Geometry: final body of the model. Coordinates: model frame, mm. Face numbers are marked on the shaded views. A direction names the side the tool comes from. Give positions to 0.01 mm unless a question says otherwise; leave off trailing zeros. Loops run counter-clockwise (first coordinate to the right, second up) from the corner with the lowest first, then second, coordinate; pieces in that order, holes last. Notation, with made-up numbers: (19, 83) -> (68, 83) arc R30 cw to (68, 111) -> close; hole circle Ø4 at (52, 2.25). An arc over 180 degrees is marked (long way). Answer in a Markdown table with one row per item. Add a question column.
1) Draft query along X for the marked faces 1, 2 and 3. Return one class per face: +X half, -X half, draft (parallel to the pull), parting line (faces both ways), or undercut.
2) Line query: line 1 (Y direction, x = 36.5, z = -34); line 2 (X direction, y = -4.5, z = -15); line 3 (Y direction, x = -7.5, z = 29.5). Output: solid intervals per line, ascending. Write a range as from..to.
3) Access query for the marked faces 4, 5 and 6. Directions: +Z, -Z, +X, -X, +Y, -Y. A direction counts if a zero-diameter tool reaches every point of the face in a straight line with its end or side. Return the directions, or none.
4) Section query D-D (x = -52.5). Give the number of separate pieces and of enclosed holes in the cut face, plus the area to 3 significant figures.
5) Section query A-A (z = 21). Return the cut outline in (x, y), plus the area to 3 significant figures.
6) Section query B-B (y = 0). Return the cut outline in (x, z), plus the area to 3 significant figures.
7) Section query C-C (x = 45.5). Return the cut outline in (y, z), plus the area to 3 significant figures.
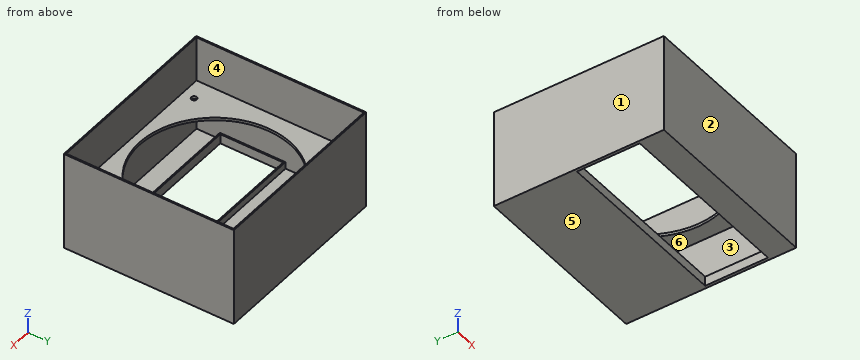
```python
from build123d import *

# Parameters (mm, degrees)
F0_W     = 134
F0_H     = 122
F0_R     = 2
F0_R_2   = 55
F1_DEPTH = 2
F0_W_2   = 136
F0_H_2   = 124
F2_DEPTH = 35
F3_W     = 136
F3_H     = 124
F3_W_2   = 134
F3_H_2   = 122
F3_W_3   = 133.8
F3_H_3   = 47.8
F3_W_4   = 131.8
F3_H_4   = 45.8
F4_DEPTH = 2
F5_DEPTH = 5


with BuildPart() as f1:
    # F0 (on Top) → F1 (new body)
    with BuildSketch(Plane.XY):
        Rectangle(F0_W, F0_H)
        with Locations((-52.5, -52.5)):
            Circle(F0_R, mode=Mode.SUBTRACT)
        with Locations((52.5, -52.5)):
            Circle(F0_R, mode=Mode.SUBTRACT)
        with Locations((-52.5, 52.5)):
            Circle(F0_R, mode=Mode.SUBTRACT)
        Circle(F0_R_2, mode=Mode.SUBTRACT)
        with Locations((52.5, 52.5)):
            Circle(F0_R, mode=Mode.SUBTRACT)
    extrude(amount=F1_DEPTH)

    # F0 (on Top) → F2 (join, symmetric)
    with BuildSketch(Plane.XY):
        Rectangle(F0_W_2, F0_H_2)
        Rectangle(F0_W, F0_H, mode=Mode.SUBTRACT)
    extrude(amount=F2_DEPTH, both=True)

    # F3 (on face) → F4 (join)
    with BuildSketch(Plane(origin=(0, 0, -35), x_dir=(1, 0, 0), z_dir=(0, 0, -1))):
        Rectangle(F3_W, F3_H)
        Rectangle(F3_W_2, F3_H_2, mode=Mode.SUBTRACT)
        Rectangle(F3_W_2, F3_H_2)
        with Locations((0, 20)):
            Rectangle(F3_W_3, F3_H_3, mode=Mode.SUBTRACT)
        with Locations((0, 20)):
            Rectangle(F3_W_3, F3_H_3)
        with Locations((0, 20)):
            Rectangle(F3_W_4, F3_H_4, mode=Mode.SUBTRACT)
    extrude(amount=F4_DEPTH)

    # F3 (on face) → F5 (join)
    with BuildSketch(Plane(origin=(0, 0, -35), x_dir=(1, 0, 0), z_dir=(0, 0, -1))):
        with Locations((0, 20)):
            Rectangle(F3_W_3, F3_H_3)
        with Locations((0, 20)):
            Rectangle(F3_W_4, F3_H_4, mode=Mode.SUBTRACT)
    extrude(amount=-F5_DEPTH)


solid = f1.part
```
Evaluation:
| question | item | result |
|---|---|---|
| 1 | face 1 | -X half |
| 1 | face 2 | draft |
| 1 | face 3 | undercut |
| 2 | line 1 | -62..-61, -43.9..-42.9, 2.9..3.9, 61..62 |
| 2 | line 2 | -68..-67, 67..68 |
| 2 | line 3 | -62..-61, 61..62 |
| 3 | face 4 | +Z |
| 3 | face 5 | -Z, +X, -X, +Y, -Y |
| 3 | face 6 | none |
| 4 | separate pieces | 4 |
| 4 | enclosed holes | 0 |
| 4 | area | 469 mm² |
| 5 | outline | (-68, -62) -> (68, -62) -> (68, 62) -> (-68, 62) -> close; hole (-67, -61) -> (67, -61) -> (67, 61) -> (-67, 61) -> close |
| 5 | area | 516 mm² |
| 6 | outline | (-68, -37) -> (-65.9, -37) -> (-65.9, -30) -> (-66.9, -30) -> (-66.9, -35) -> (-67, -35) -> (-67, 0) -> (-55, 0) -> (-55, 2) -> (-67, 2) -> (-67, 35) -> (-68, 35) -> close; (55, 0) -> (67, 0) -> (67, -35) -> (66.9, -35) -> (66.9, -30) -> (65.9, -30) -> (65.9, -37) -> (68, -37) -> (68, 35) -> (67, 35) -> (67, 2) -> (55, 2) -> close |
| 6 | area | 206 mm² |
| 7 | outline | (-62, -37) -> (-42.9, -37) -> (-42.9, -30) -> (-43.9, -30) -> (-43.9, -35) -> (-61, -35) -> (-61, 0) -> (-30.9, 0) -> (-30.9, 2) -> (-61, 2) -> (-61, 35) -> (-62, 35) -> close; (2.9, -37) -> (62, -37) -> (62, 35) -> (61, 35) -> (61, 2) -> (30.9, 2) -> (30.9, 0) -> (61, 0) -> (61, -35) -> (3.9, -35) -> (3.9, -30) -> (2.9, -30) -> close |
| 7 | area | 427 mm² |
